```python
from build123d import *

# Parameters (mm, degrees)
F1_DEPTH = 1
F4_DEPTH = 25


with BuildPart() as f1:
    # F0 (on Front) → F1 (new body)
    with BuildSketch(Plane.XZ):
        with BuildLine():
            Line((-32.070443, 0), (0, 0))
            Line((0, 0), (32.070443, 0))
            ThreePointArc((32.070443, 0), (36.842031, 1.211829), (40.457149, 4.55361))
            Line((40.457149, 4.55361), (90.350609, 81.382801))
            ThreePointArc((90.350609, 81.382801), (91.552101, 83.989038), (91.963904, 86.829192))
            Line((91.963904, 86.829192), (91.963904, 108.867057))
            ThreePointArc((91.963904, 108.867057), (89.034971, 115.938125), (81.963904, 118.867057))
            Line((81.963904, 118.867057), (-81.963904, 118.867057))
            ThreePointArc((-81.963904, 118.867057), (-89.034971, 115.938125), (-91.963904, 108.867057))
            Line((-91.963904, 108.867057), (-91.963904, 86.829192))
            ThreePointArc((-91.963904, 86.829192), (-91.552101, 83.989038), (-90.350609, 81.382801))
            Line((-90.350609, 81.382801), (-40.457149, 4.55361))
            ThreePointArc((-40.457149, 4.55361), (-36.842031, 1.211829), (-32.070443, 0))
        make_face()
    extrude(amount=F1_DEPTH)


with BuildPart() as f2_1:
    # F2: copy of F1
    add(f1.part)


with BuildPart() as f4_tool:
    # F3 (on face) → F4 (new body)
    with BuildSketch(Plane.XZ.offset(1)):
        with BuildLine():
            Line((76.963904, 108.867057), (-76.963904, 108.867057))
            ThreePointArc((-76.963904, 108.867057), (-80.499437, 107.402591), (-81.963904, 103.867057))
            Line((-81.963904, 103.867057), (-81.963904, 91.829192))
            ThreePointArc((-81.963904, 91.829192), (-80.499437, 88.293658), (-76.963904, 86.829192))
            Line((-76.963904, 86.829192), (76.963904, 86.829192))
            ThreePointArc((76.963904, 86.829192), (80.499437, 88.293658), (81.963904, 91.829192))
            Line((81.963904, 91.829192), (81.963904, 103.867057))
            ThreePointArc((81.963904, 103.867057), (80.499437, 107.402591), (76.963904, 108.867057))
        make_face()
    extrude(amount=-F4_DEPTH)


with BuildPart() as f1_1:
    add(f1.part)

    # F4: cut by f4_tool
    add(f4_tool.part, mode=Mode.SUBTRACT)


with BuildPart() as f2_1_1:
    add(f2_1.part)

    # F4: cut by f4_tool
    add(f4_tool.part, mode=Mode.SUBTRACT)


solid = f1_1.part
```
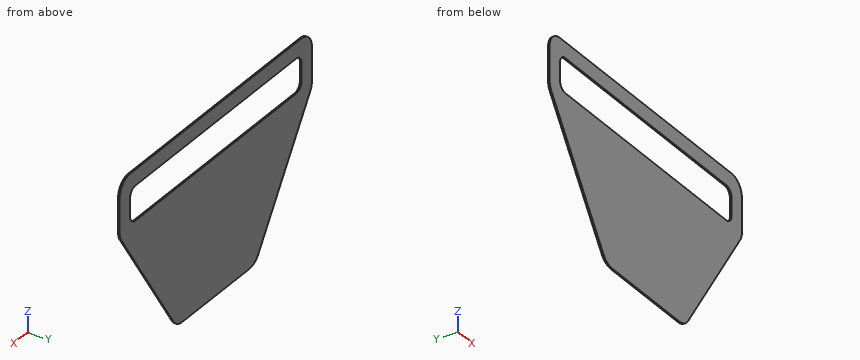
Check sheet for the modelled part. Datum: model origin and axes. Units: mm. Coordinates: 2 decimals unless noted, no trailing zeros. Write each loop counter-clockwise with the first axis right and the second up, starting at its lowest first coordinate (ties: lowest second). Pieces come first, ordered by that corner, then holes. Notation, with made-up numbers: (79, 89) - (112, 89) arc R22 cw to (112, 127) - close; hole circle Ø7 at (88.25, -8). An arc over 180 degrees is marked (long way). One line per question, with ' | ' between items.
Item 1: Sectioned sample at A-A on x = -29. Record the boundary of the cut face in (y, z), plus the area to 3 significant figures.
Determined:
outline: (-1, 0) - (0, 0) - (0, 86.83) - (-1, 86.83) - close; (-1, 108.87) - (0, 108.87) - (0, 118.87) - (-1, 118.87) - close | area: 96.8 mm2
Item 2: Sectioned sample at B-B on y = -0.6. Record the boundary of the cut face in (x, z).
Determined:
outline: (-91.96, 86.83) arc R10 ccw to (-90.35, 81.38) - (-40.46, 4.55) arc R10 ccw to (-32.07, 0) - (32.07, 0) arc R10 ccw to (40.46, 4.55) - (90.35, 81.38) arc R10 ccw to (91.96, 86.83) - (91.96, 108.87) arc R10 ccw to (81.96, 118.87) - (-81.96, 118.87) arc R10 ccw to (-91.96, 108.87) - close; hole (-81.96, 91.83) arc R5 ccw to (-76.96, 86.83) - (76.96, 86.83) arc R5 ccw to (81.96, 91.83) - (81.96, 103.87) arc R5 ccw to (76.96, 108.87) - (-76.96, 108.87) arc R5 ccw to (-81.96, 103.87) - close
Item 3: Thickness scan on line 1 (Z direction, x = 4.5, y = -0.85); line 2 (X direction, y = -0.6, z = 103); line 3 (Z direction, x = 63, y = -0.85). Record the ranges inside material, lowest first. Write a range as [from, to].
Determined:
line 1: z = [0, 86.83], [108.87, 118.87] | line 2: x = [-91.96, -81.96], [81.96, 91.96] | line 3: z = [39.27, 86.83], [108.87, 118.87]
Item 4: Sectioned sample at D-D on z = 16.5. Record the boundary of the cut face in (x, y), plus the area to 3 significant figures.
Determined:
outline: (-48.22, -1) - (48.22, -1) - (48.22, 0) - (-48.22, 0) - close | area: 96.4 mm2
Item 5: Sectioned sample at C-C on z = 107. Record the boundary of the cut face in (x, y).
Determined:
outline: (-91.96, -1) - (-80.86, -1) - (-80.86, 0) - (-91.96, 0) - close; (80.86, -1) - (91.96, -1) - (91.96, 0) - (80.86, 0) - close
